```python
from build123d import *

# Parameters (mm, degrees)
BOSS_EXTRUDE1_DEPTH      = 5
BOSS_EXTRUDE1_DEPTH_BACK = 0.093151617
SKETCH1_W                = 182.5752
SKETCH1_H                = 73.4568
SKETCH2_R                = 3.416363386
BOSS_EXTRUDE2_DEPTH      = 7
SKETCH3_R                = 1.85
BOSS_EXTRUDE3_DEPTH      = 5
SKETCH4_W                = 191.110733906
SKETCH4_H                = 81.992333906
SKETCH4_W_2              = 182.5752
SKETCH4_H_2              = 73.4568
BOSS_EXTRUDE4_DEPTH      = 12
SKETCH5_W                = 191.110733906
SKETCH5_H                = 81.992333906
BOSS_EXTRUDE5_DEPTH      = 5.093151617
SKETCH7_W                = 182.5752
SKETCH7_H                = 73.4568
BOSS_EXTRUDE7_DEPTH      = 5
CUT_EXTRUDE1_START       = -2
CUT_EXTRUDE1_DEPTH       = 6


with BuildPart() as part:
    # Sketch1 → Boss-Extrude1 (new, two sides: drawn at the far end of the back side and taken through both)
    with BuildSketch(Plane.XY.offset(-BOSS_EXTRUDE1_DEPTH_BACK)):
        with Locations((-10.337299282, 18.489677755)):
            Rectangle(SKETCH1_W, SKETCH1_H)
    extrude(amount=BOSS_EXTRUDE1_DEPTH + BOSS_EXTRUDE1_DEPTH_BACK)

    # Sketch2 → Boss-Extrude2 (add)
    with BuildSketch(Plane.XY.offset(5)):
        with Locations((-97.941899282, 50.950877755)):
            Circle(SKETCH2_R)
        with Locations((76.810100718, 50.950877755)):
            Circle(SKETCH2_R)
        with Locations((76.810100718, -14.276322245)):
            Circle(SKETCH2_R)
        with Locations((-97.941899282, -14.276322245)):
            Circle(SKETCH2_R)
    extrude(amount=BOSS_EXTRUDE2_DEPTH)

    # Sketch3 → Boss-Extrude3 (add)
    with BuildSketch(Plane.XY.offset(12)):
        with Locations((-97.941899282, 50.950877755)):
            Circle(SKETCH3_R)
        with Locations((-97.941899282, -14.276322245)):
            Circle(SKETCH3_R)
        with Locations((76.810100718, -14.276322245)):
            Circle(SKETCH3_R)
        with Locations((76.810100718, 50.950877755)):
            Circle(SKETCH3_R)
    extrude(amount=BOSS_EXTRUDE3_DEPTH)



with BuildPart() as body_2:
    # Sketch4 → Boss-Extrude4 (new body)
    with BuildSketch(Plane.XY.offset(5)):
        with Locations((-11.069532329, 19.221910802)):
            Rectangle(SKETCH4_W, SKETCH4_H)
        with Locations((-10.337299282, 18.489677755)):
            Rectangle(SKETCH4_W_2, SKETCH4_H_2, mode=Mode.SUBTRACT)
    extrude(amount=BOSS_EXTRUDE4_DEPTH)


with BuildPart() as part_1:
    add(part.part)

    add(body_2.part)  # Boss-Extrude5 merges body 2
    # Sketch5 → Boss-Extrude5 (add)
    with BuildSketch(Plane(origin=(0, 0, 5), x_dir=(-1, 0, 0), z_dir=(0, 0, -1))):
        with Locations((11.069532329, 19.221910802)):
            Rectangle(SKETCH5_W, SKETCH5_H)
    extrude(amount=BOSS_EXTRUDE5_DEPTH)

    # Sketch7 → Boss-Extrude7 (add)
    with BuildSketch(Plane.XY.offset(5)):
        with Locations((-10.337299282, 18.489677755)):
            Rectangle(SKETCH7_W, SKETCH7_H)
    extrude(amount=BOSS_EXTRUDE7_DEPTH)

    # Sketch6 → Cut-Extrude1 (cut)
    with BuildSketch(Plane(origin=(0, 0, -0.093151617), x_dir=(-1, 0, 0), z_dir=(0, 0, -1)).offset(CUT_EXTRUDE1_START)):
        Polygon((-84.485834624, 34.360708249), (-84.485834624, 4.083113354), (-66.229962778, 4.083113354), (-66.229962778, 0.271521895), (-63.510633591, 0.271521895), (-56.864299396, 4.083113354), (-56.864299396, 34.360708249), (-63.510633591, 38.172299708), (-66.229962778, 38.172299708), (-66.229962778, 34.360708249), align=None)
    cut_extrude1 = extrude(amount=-CUT_EXTRUDE1_DEPTH, mode=Mode.SUBTRACT)

    # Mirror1: Cut-Extrude1 across plane
    add(cut_extrude1.mirror(Plane(origin=(-11.069532329, 0, 0), x_dir=(0, 0, 1), z_dir=(1, 0, 0))), mode=Mode.SUBTRACT)


solid = part_1.part
```
Geometry check sheet. Reference: the model listing, model coordinates, mm. A direction names the side the tool comes from. Round coordinates to 2 decimals unless told otherwise and drop trailing zeros. Write each loop counter-clockwise with the first axis right and the second up, starting at its lowest first coordinate (ties: lowest second). Pieces come first, ordered by that corner, then holes. Notation, with made-up numbers: (-11.5, -35.5) -> (21.5, -35.5) arc R23 cw to (21.5, -2.5) -> close; hole circle Ø4 at (-27, -16). An arc over 180 degrees is marked (long way). Put each result on its own line as item: value.
1) Access from +Z, -Z, +X, -X, +Y, -Y to the whole of each face (thin tool, end or side, straight path). Record for faces 3 (the face through (78, 49, 12)), 4 (the face through (75, 34.361, 5)), 5 (the face through (-98, 4.083, 5)).
Recorded:
face 3: +Z
face 4: +X
face 5: -X
2) Cross-section at B-B, the plane z = 4.5. Enter the section's corners in (x, y).
Recorded:
outline: (-106.62, -21.77) -> (84.49, -21.77) -> (84.49, 4.08) -> (66.23, 4.08) -> (66.23, 0.27) -> (63.51, 0.27) -> (56.86, 4.08) -> (56.86, 34.36) -> (63.51, 38.17) -> (66.23, 38.17) -> (66.23, 34.36) -> (84.49, 34.36) -> (84.49, 60.22) -> (-106.62, 60.22) -> (-106.62, 34.36) -> (-88.37, 34.36) -> (-88.37, 38.17) -> (-85.65, 38.17) -> (-79, 34.36) -> (-79, 4.08) -> (-85.65, 0.27) -> (-88.37, 0.27) -> (-88.37, 4.08) -> (-106.62, 4.08) -> close
3) Depth check by flat-ended pin: P1, Ø5, axis at x = 33.5, y = 2, coming from the +Z side; P2, Ø6.5, axis at y = 21.5, z = 4.5, coming from the +X side; P3, Ø5, axis at y = 16, z = 4.5, coming from the -X side. Enter the tip coordinate at first touch or a pass-through.
Recorded:
P1: stops at z = 10
P2: stops at x = 84.49
P3: stops at x = -79
4) Thickness scan on probe 1 along X at (y, z) = (18, 15.5); probe 2 along Y at (x, z) = (-44, 13); probe 3 along Z at (x, y) = (-30, -14). Record the ranges inside material, lowest first. Write a range as from..to.
Recorded:
probe 1: x = -106.62..-101.62, 80.95..84.49
probe 2: y = -21.77..-18.24, 55.22..60.22
probe 3: z = -0.09..10
5) Cross-section at A-A, the plane y = 41. Enter the section's corners in (x, z).
Recorded:
outline: (-106.62, -0.09) -> (84.49, -0.09) -> (84.49, 17) -> (80.95, 17) -> (80.95, 10) -> (-101.62, 10) -> (-101.62, 17) -> (-106.62, 17) -> close
6) Cross-section at C-C, the plane z = 15. Enter the section's corners in (x, y), plus the area to 3 significant figures.
Recorded:
outline: (-106.62, -21.77) -> (84.49, -21.77) -> (84.49, 60.22) -> (-106.62, 60.22) -> close; circle Ø3.7 at (-97.94, -14.28); circle Ø3.7 at (-97.94, 50.95); circle Ø3.7 at (76.81, -14.28); circle Ø3.7 at (76.81, 50.95); hole (-101.62, -18.24) -> (80.95, -18.24) -> (80.95, 55.22) -> (-101.62, 55.22) -> close
area: 2,300 mm2
7) Release check for a two-part mould opening along Y. For faces 1 (the face through (-106.625, 19, 9)), 2 (the face through (71, 19, 7.907)) record: pulls with the +Y half, pulls with the -Y half, needs draft (parallel to the pull), parting line crosses it, or undercut.
Recorded:
face 1: needs draft
face 2: undercut
8) Cross-section at D-D, the plane x = -44. Enter the section's corners in (y, z).
Recorded:
outline: (-21.77, -0.09) -> (60.22, -0.09) -> (60.22, 17) -> (55.22, 17) -> (55.22, 10) -> (-18.24, 10) -> (-18.24, 17) -> (-21.77, 17) -> close
